```python
from build123d import *

# Parameters (mm, degrees)
F1_DEPTH = 19.05


with BuildPart() as f1:
    # F0 (on Front) → F1 (new body)
    with BuildSketch(Plane.XZ):
        with BuildLine():
            ThreePointArc((24.339379, -7.263239), (22.4, 0), (24.339379, 7.263239))
            ThreePointArc((24.339379, 7.263239), (22.458654, 8.174281), (23.313766, 10.081087))
            ThreePointArc((23.313766, 10.081087), (17.159396, 14.398442), (13.976326, 21.209015))
            ThreePointArc((13.976326, 21.209015), (11.95, 20.698007), (11.379383, 22.708361))
            ThreePointArc((11.379383, 22.708361), (3.889719, 22.059694), (-2.926405, 25.230857))
            ThreePointArc((-2.926405, 25.230857), (-2.914604, 25.122772), (-2.910664, 25.014117))
            ThreePointArc((-2.910664, 25.014117), (-4.257881, 23.521918), (-5.87954, 24.71014))
            ThreePointArc((-5.87954, 24.71014), (-11.2, 19.398969), (-18.459839, 17.446901))
            ThreePointArc((-18.459839, 17.446901), (-18.088855, 16.940591), (-17.957529, 16.326805))
            ThreePointArc((-17.957529, 16.326805), (-18.803598, 14.976852), (-20.387361, 15.14977))
            ThreePointArc((-20.387361, 15.14977), (-21.049115, 7.661251), (-25.355709, 1.499346))
            ThreePointArc((-25.355709, 1.499346), (-24.323794, 1.044883), (-23.9, 0))
            ThreePointArc((-23.9, 0), (-24.323794, -1.044883), (-25.355709, -1.499346))
            ThreePointArc((-25.355709, -1.499346), (-21.049115, -7.661251), (-20.387361, -15.14977))
            ThreePointArc((-20.387361, -15.14977), (-18.803598, -14.976852), (-17.957529, -16.326805))
            ThreePointArc((-17.957529, -16.326805), (-18.088855, -16.940591), (-18.459839, -17.446901))
            ThreePointArc((-18.459839, -17.446901), (-11.2, -19.398969), (-5.87954, -24.71014))
            ThreePointArc((-5.87954, -24.71014), (-4.257881, -23.521918), (-2.910664, -25.014117))
            ThreePointArc((-2.910664, -25.014117), (-2.914604, -25.122772), (-2.926405, -25.230857))
            ThreePointArc((-2.926405, -25.230857), (3.889719, -22.059694), (11.379383, -22.708361))
            ThreePointArc((11.379383, -22.708361), (11.95, -20.698007), (13.976326, -21.209015))
            ThreePointArc((13.976326, -21.209015), (17.159396, -14.398442), (23.313766, -10.081087))
            ThreePointArc((23.313766, -10.081087), (22.458654, -8.174281), (24.339379, -7.263239))
        make_face()
    extrude(amount=F1_DEPTH)


solid = f1.part
```
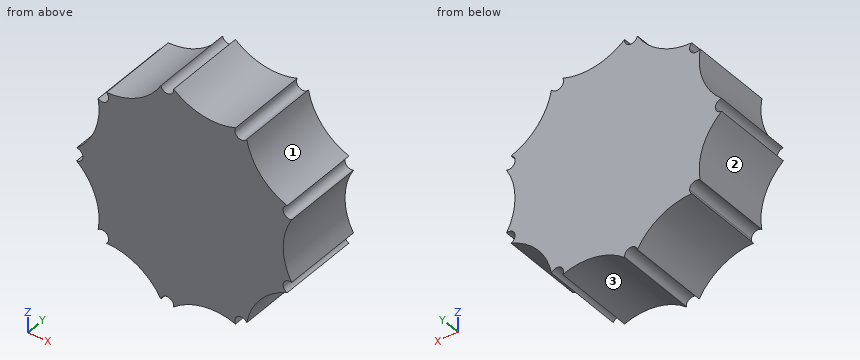
The model under review builds one solid part; all positions refer to its coordinate system, in mm. Face numbers are marked on the shaded views. Round coordinates to 2 decimals unless told otherwise and drop trailing zeros. Write each loop counter-clockwise with the first axis right and the second up, starting at its lowest first coordinate (ties: lowest second). Pieces come first, ordered by that corner, then holes. Notation, with made-up numbers: (80.5, 25.5) -> (132.5, 25.5) arc R13 cw to (132.5, 42.5) -> close; hole circle Ø2 at (62.25, -17). An arc over 180 degrees is marked (long way). Use CSV: the item, a comma, the result in double quotes.
Q1. Mouldability with a two-part tool opening along X and no side actions: class the marked faces 1, 2 and 3 as released by +X, released by -X, zero draft, split by the parting line, or undercut.
Checks:
face 1,"released by +X"
face 2,"released by -X"
face 3,"undercut"
Q2. Consider section C-C (z = 3.5). Give the boundary of the cut face in (x, y).
Checks:
outline,"(-23.4, -19.05) -> (22.83, -19.05) -> (22.83, 0) -> (-23.4, 0) -> close"
Q3. For pin 1 Ø10 at (y, z) = (-14.5, -17) entering from +X; pin 2 Ø8 at (y, z) = (-16, 17.5) entering from +X; pin 3 Ø1.5 at (x, y) = (3, -5) entering from -Z, all flat-tipped, find the tip position at first contact; note any pin that passes through.
Checks:
pin 1,"x = 19.72"
pin 2,"x = 17.98"
pin 3,"z = -22.45"
Q4. Consider section A-A (y = -9.25). Give the boundary of the cut face in (x, z).
Checks:
outline,"(-25.36, -1.5) arc R14.57 cw to (-20.39, -15.15) arc R1.5 cw to (-17.96, -16.33) arc R1.5 cw to (-18.46, -17.45) arc R14.57 cw to (-5.88, -24.71) arc R1.5 cw to (-2.91, -25.01) arc R1.5 cw to (-2.93, -25.23) arc R14.57 cw to (11.38, -22.71) arc R1.5 cw to (13.98, -21.21) arc R14.57 cw to (23.31, -10.08) arc R1.5 cw to (24.34, -7.26) arc R14.57 cw to (24.34, 7.26) arc R1.5 cw to (23.31, 10.08) arc R14.57 cw to (13.98, 21.21) arc R1.5 cw to (11.38, 22.71) arc R14.57 cw to (-2.93, 25.23) arc R1.5 cw to (-2.91, 25.01) arc R1.5 cw to (-5.88, 24.71) arc R14.57 cw to (-18.46, 17.45) arc R1.5 cw to (-17.96, 16.33) arc R1.5 cw to (-20.39, 15.15) arc R14.57 cw to (-25.36, 1.5) arc R1.5 cw to start"
Q5. To check wall thickness, follow probe 1 along Z at (x, y) = (6.5, -9); probe 2 along Z at (x, y) = (7, -17.5); probe 3 along X at (y, z) = (-11.5, 2). State the ranges of each line that lie inside material, in increasing order. Write a range as [from, to].
Checks:
probe 1,"[-21.84, 21.84]"
probe 2,"[-21.85, 21.85]"
probe 3,"[-24.79, 22.54]"
Q6. Consider section B-B (x = 12.7). Give the boundary of the cut face in (y, z), then the cut area to 3 significant figures.
Checks:
outline,"(-19.05, -20.5) -> (0, -20.5) -> (0, 20.5) -> (-19.05, 20.5) -> close"
area,"781 mm²"
